Geometry check sheet. Reference: drawing and pictorial views, mm from the part's lowest x, y, z. A direction names the side the tool comes from. Give positions to 0.01 mm unless a question says otherwise; leave off trailing zeros. Order: outer loops, then holes, each group sorted by start corner. A loop starts at its lowest first (then second) coordinate and runs counter-clockwise, first axis right, second up.
Item 1: Sectioned sample at A-A on x = 19. Record the boundary of the cut face in (y, z), and give its area (3 significant figures).
Item 2: Sectioned sample at D-D on x = 24.5. Record the boundary of the cut face in (y, z), and give its area (3 significant figures).
Item 3: Access from +Z, -Z, +X, -X, +Y, -Y to the whole of each face (thin tool, end or side, straight path). Record for the marked faces 1, 2 and 3.
Item 4: Sectioned sample at B-B on z = 7.5. Record the boundary of the cut face in (x, y).
Item 5: Release check for a two-part mould opening along Y. For the marked faces 4, 5 and 6 record: released by +Y, released by -Y, zero draft, split by the parting line, or undercut.
Item 6: Gauge pin test, flat ends, axial feed: P1, Ø3, axis at x = 27.5, y = 5.5, coming from the +Z side; P2, Ø1.5, axis at y = 22, z = 28.5, coming from the -X side; P3, Ø12, axis at y = 33.5, z = 18.5, coming from the +X side. Record the tip position at first contact, or that the pin passes through.
Item 7: Material ranges on line 1 along Y through (x, z) = (19, 16.5); line 2 along Y through (x, z) = (19, 35.9); line 3 along Z through (x, y) = (27.5, 5.5), recorded low to high.
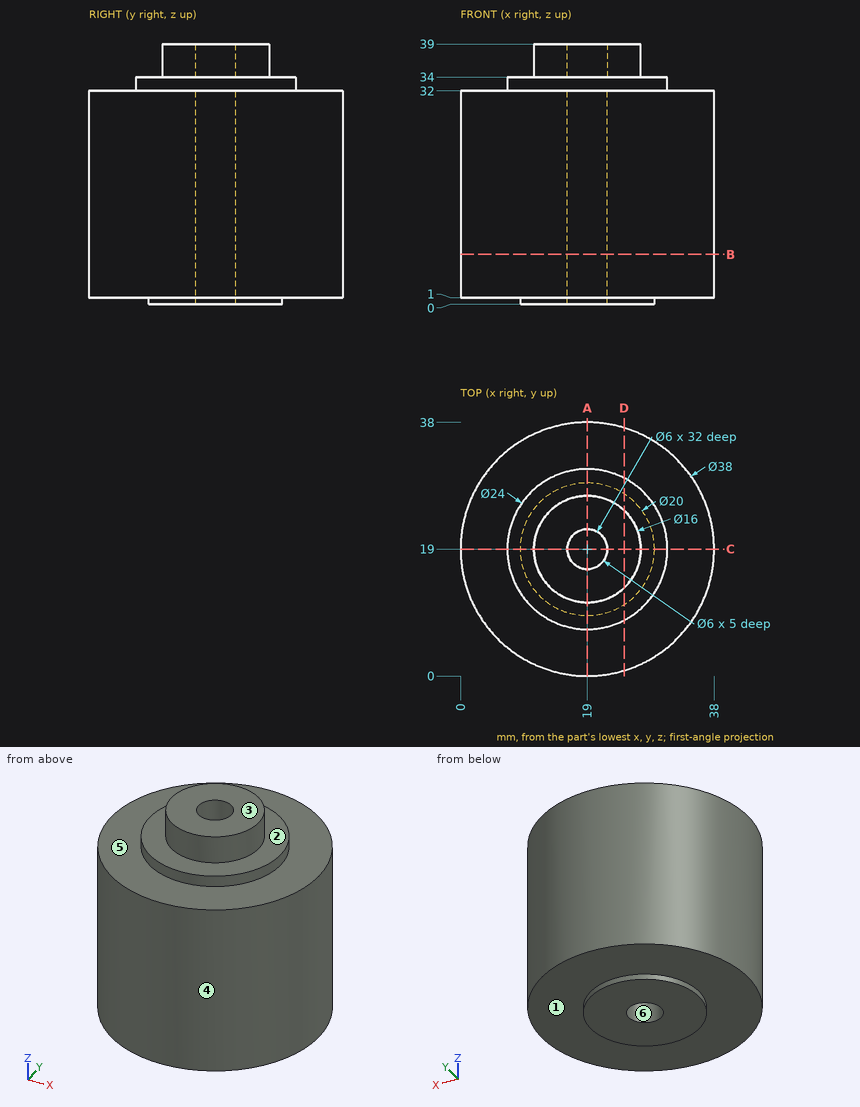
Report:
1. outline: (0, 1) - (9, 1) - (9, 0) - (16, 0) - (16, 32) - (22, 32) - (22, 0) - (29, 0) - (29, 1) - (38, 1) - (38, 32) - (31, 32) - (31, 34) - (27, 34) - (27, 39) - (22, 39) - (22, 34) - (16, 34) - (16, 39) - (11, 39) - (11, 34) - (7, 34) - (7, 32) - (0, 32) - close
1. area: 1,100 mm2
2. outline: (0.81, 1) - (10.65, 1) - (10.65, 0) - (27.35, 0) - (27.35, 1) - (37.19, 1) - (37.19, 32) - (29.67, 32) - (29.67, 34) - (24.81, 34) - (24.81, 39) - (13.19, 39) - (13.19, 34) - (8.33, 34) - (8.33, 32) - (0.81, 32) - close
2. area: 1,250 mm2
3. face 1: -Z
3. face 2: +Z
3. face 3: +Z, +X, -X, +Y, -Y
4. outline: circle Ø38 at (19, 19); hole circle Ø6 at (19, 19)
5. face 4: split by the parting line
5. face 5: zero draft
5. face 6: undercut
6. P1: stops at z = 32
6. P2: stops at x = 0.13
6. P3: stops at x = 35.99
7. line 1: y = 0 to 16, 22 to 38
7. line 2: y = 11 to 16, 22 to 27
7. line 3: z = 1 to 32
